Autodesk Inventor part; units mm, degrees
ref_plane "YZ Plane" through (0, 0, 0) normal (1, 0, 0) x (0, 1, 0)
ref_plane "XZ Plane" through (0, 0, 0) normal (0, 1, 0) x (-1, 0, 0)
ref_plane "XY Plane" through (0, 0, 0) normal (0, 0, 1) x (1, 0, 0)
sketch "스케치1" plane through (0, 0, 0) normal (0, 0, 1) x (1, 0, 0)
  circle A0 centre (0, 0) radius 2.5
  circle A1 centre (0, 0) radius 5
  line L0 (0, -5) -> (25, -5)
  line L1 (25, -5) -> (25, 5)
  line L2 (25, 5) -> (20, 5)
  line L3 (20, 5) -> (16, 1)
  line L4 (16, 1) -> (6, 1)
  line L5 (6, 1) -> (6, 5)
  line L6 (6, 5) -> (0, 5)
  dimension "d0" = 5
  dimension "d1" = 10
  dimension "d2" = 25
  dimension "d3" = 10
  dimension "d4" = 90
  dimension "d5" = 5
  dimension "d6" = 90
  dimension "d7" = 10
  dimension "d8" = 4
  dimension "d9" = 4
extrude "돌출1" add sketch "스케치1" along normal mid plane 17
extrude "돌출2" add sketch "스케치1" along normal mid plane 32 contours A0
sketch "스케치2" plane through (0, 0, 0) normal (0, 0, 1) x (1, 0, 0)
  line L0 (5, 11.5318) -> (29.4408, 11.5318)
  line L1 (29.4408, 11.5318) -> (29.4408, -9.0869)
  line L2 (29.4408, -9.0869) -> (5, -9.0869)
  line L3 (5, -9.0869) -> (5, 11.5318)
  line L4 (25, 5) -> (25, -5)
  point P0 (0, 0)
  dimension "d14" = 20
extrude "돌출3" cut sketch "스케치2" along normal mid plane 8
chamfer "모따기1" distance 3 angle 45 2 edges at (25, -5, 6.25) (25, -5, -6.25)
properties part number "10-2"
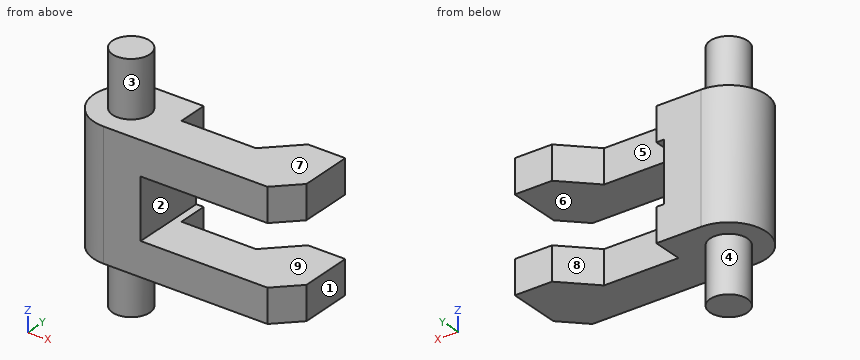
Work out the finished part from the listing and answer in its coordinate system (mm). Face numbers are marked on the shaded views. A direction names the side the tool comes from. Give positions to 0.01 mm unless a question says otherwise; leave off trailing zeros. Write each loop counter-clockwise with the first axis right and the second up, starting at its lowest first coordinate (ties: lowest second). Pieces come first, ordered by that corner, then holes.
Q1. For a pull along Z with two mould halves and no side action, classify the marked faces 6, 7, 8 and 9 as released by +Z, released by -Z, zero draft, split by the parting line, or undercut.
Answer:
face 6: undercut
face 7: released by +Z
face 8: zero draft
face 9: undercut
Q2. The part is cut by section C-C on z = -6.5. Give the vertices of the cut face in (x, y), and give its area (3 significant figures).
Answer:
outline: (0, -5) - (22, -5) - (25, -2) - (25, 5) - (20, 5) - (16, 1) - (6, 1) - (6, 5) - (0, 5) arc R5 ccw to start
area: 237 mm2
Q3. Given pin 1 (2.5 mm diameter, centred on y = 0, z = -1, fed in from +X); pin 2 (3 mm diameter, centred on x = 20, y = 1.5, fed in from -Z); pin 3 (5 mm diameter, centred on y = 2, z = -11.5, fed in from +X); pin 4 (12 mm diameter, centred on x = 0.5, z = -12, fed in from -Y), each flat-ended and moving along its own axis, determine where each tip first touches the part or whether it passes through.
Answer:
pin 1: stops at x = 5
pin 2: stops at z = -8.5
pin 3: stops at x = 2.5
pin 4: stops at y = -5
Q4. The part is cut by section B-B on y = -3. Give the vertices of the cut face in (x, z).
Answer:
outline: (-4, -8.5) - (24, -8.5) - (24, -4) - (5, -4) - (5, 4) - (24, 4) - (24, 8.5) - (-4, 8.5) - close
Q5. A tool of negligible diameter and unlimited length cuts with its end or side. For the marked faces 1, 2, 3, 4 and 5, from which of +Z, -Z, +X, -X, +Y, -Y can it reach the whole face along a straight path? Write none if from no direction.
Answer:
face 1: +Z, -Z, +X, +Y, -Y
face 2: +X, +Y, -Y
face 3: +Z
face 4: -Z
face 5: +Z, -Z, +Y
Q6. The part is cut by section A-A on x = 18.5. Give the vertices of the cut face in (y, z), and give its area (3 significant figures).
Answer:
outline: (-5, -8.5) - (3.5, -8.5) - (3.5, -4) - (-5, -4) - close; (-5, 4) - (3.5, 4) - (3.5, 8.5) - (-5, 8.5) - close
area: 76.5 mm2
Q7. Straight lines are drawn through the part: L1, parallel to Z at x = 13.5, y = -2.5; L2, parallel to Z at x = -2.25, y = -2.25; L3, parallel to X at y = 0.25, z = 6. For each, find the intervals that lie inside material, in ascending order.
Answer:
L1: z = -8.5 to -4, 4 to 8.5
L2: z = -8.5 to 8.5
L3: x = -4.99 to 25
Q8. The part is cut by section D-D on x = 7.75. Give the vertices of the cut face in (y, z), and give its area (3 significant figures).
Answer:
outline: (-5, -8.5) - (1, -8.5) - (1, -4) - (-5, -4) - close; (-5, 4) - (1, 4) - (1, 8.5) - (-5, 8.5) - close
area: 54.0 mm2
